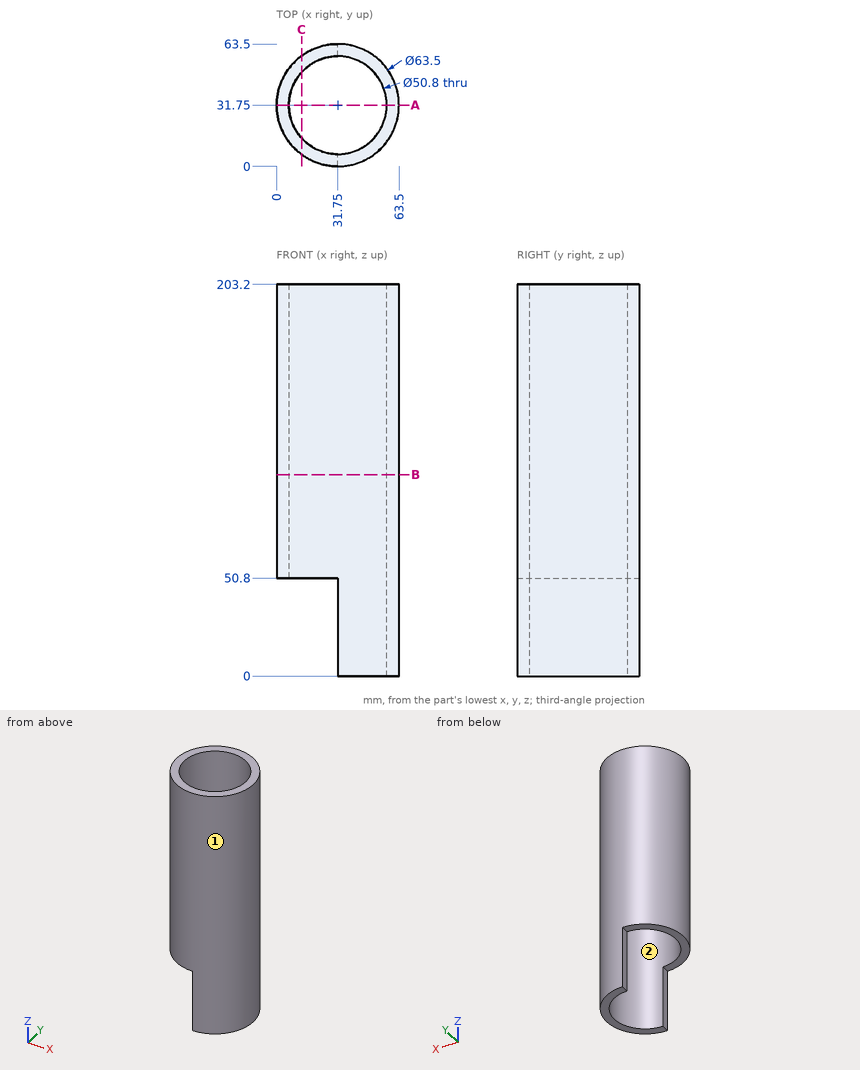
Drawing for the job (mm, zero at the part's lowest x, y, z). Round coordinates to 2 decimals unless told otherwise and drop trailing zeros. Order: outer loops, then holes, each group sorted by start corner. A loop starts at its lowest first (then second) coordinate and runs counter-clockwise, first axis right, second up. Notation, with made-up numbers: (55, 30) -> (87, 30) arc R17 cw to (87, 50) -> close; hole circle Ø11 at (25, -25.5). An arc over 180 degrees is marked (long way). Write item = value, one per line. Start each with the question number.
(1) Pin check, flat tips, straight feed: P1, Ø5, axis at y = 23, z = 180, coming from the -X side; P2, Ø4, axis at x = 26, z = 64.5, coming from the +Y side; P3, Ø3, axis at y = 47.5, z = 140, coming from the +X side. Stop position of each tip, or through.
(2) Cut at B-B, the plane z = 104.5. List the corners of the cut face in (x, y).
(3) Probe line 1 (X direction, y = 31.75, z = 121.5); line 2 (Y direction, x = 31, z = 92); line 3 (X direction, y = 35.5, z = 126). List the from-to ranges inside material, lowest first. Write a range as [from, to].
(4) Pull direction X, two halves, no side cores. Call the marked faces 1 and 2: released by +X, released by -X, zero draft, split by the parting line, or undercut.
(5) Cut at A-A, the plane y = 31.75. List the corners of the cut face in (x, z).
(6) Cut at C-C, the plane x = 13. List the corners of the cut face in (y, z), then the cut area to 3 significant figures.
Model answer:
q1.P1 = 0.62
q1.P2 = 63.28
q1.P3 = 60.12
q2.outline = circle Ø63.5 at (31.75, 31.75); hole circle Ø50.8 at (31.75, 31.75)
q3.line_1 = [0, 6.35], [57.15, 63.5]
q3.line_2 = [0.01, 6.36], [57.14, 63.49]
q3.line_3 = [0.22, 6.63], [56.87, 63.28]
q4.face_1 = split by the parting line
q4.face_2 = undercut
q5.outline = (0, 50.8) -> (6.35, 50.8) -> (6.35, 203.2) -> (0, 203.2) -> close; (57.15, 0) -> (63.5, 0) -> (63.5, 203.2) -> (57.15, 203.2) -> close
q6.outline = (6.13, 50.8) -> (14.62, 50.8) -> (14.62, 203.2) -> (6.13, 203.2) -> close; (48.88, 50.8) -> (57.37, 50.8) -> (57.37, 203.2) -> (48.88, 203.2) -> close
q6.area = 2,590 mm2
